Geometry: final body of the model. Coordinates: model frame, mm. Face numbers are marked on the shaded views. Give positions to 0.01 mm unless a question says otherwise; leave off trailing zeros. Write each loop counter-clockwise with the first axis right and the second up, starting at its lowest first coordinate (ties: lowest second). Pieces come first, ordered by that corner, then holes. Notation, with made-up numbers: (86, -13) - (132, -13) arc R28 ccw to (132, 17) - close; hole circle Ø2 at (4, 86.5). An arc over 180 degrees is marked (long way). Use CSV: the item, a comma, the result in double quotes. Start each with the question number.
(1) Section A-A on y = 0. Output: boundary loops of the cut face in (x, z), and give its area (3 significant figures).
(2) Section D-D on z = 87. Output: boundary loops of the cut face in (x, y).
(3) Section B-B on z = -21.5. Output: boundary loops of the cut face in (x, y).
(4) First-contact query: pin 1 Ø5 at (y, z) = (-79.5, -11.5) entering from -X; pin 2 Ø6 at (y, z) = (-25, 66.5) entering from +X; pin 3 Ø6 at (y, z) = (50, 42.5) entering from +X. Flat tips, straight axial feed; report the tip coordinate or a pass-through.
(5) Line query: probe 1 along Y at (x, z) = (0, -23); probe 2 along Y at (x, z) = (0, 63). Output: solid intervals per line, ascending. Write a range as [from, to].
(6) Draft query along Y for the marked faces 1, 2 and 3. Return one class per face: released by +Y, released by -Y, zero draft, split by the parting line, or undercut.
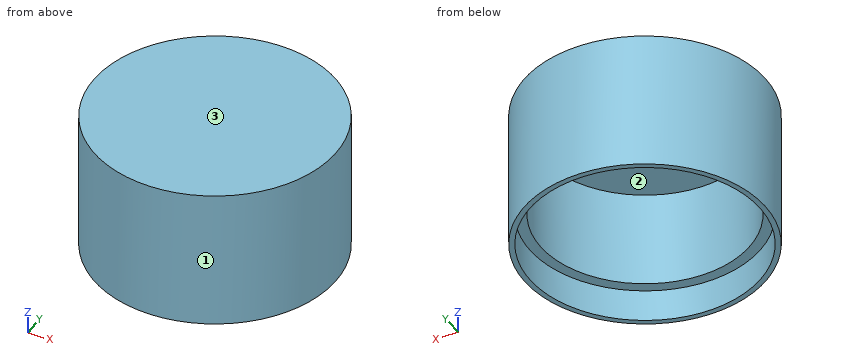
Autodesk Inventor part; units mm, degrees
ref_plane "YZ Plane" through (0, 0, 0) normal (1, 0, 0) x (0, 1, 0)
ref_plane "XZ Plane" through (0, 0, 0) normal (0, 1, 0) x (-1, 0, 0)
ref_plane "XY Plane" through (0, 0, 0) normal (0, 0, 1) x (1, 0, 0)
sketch "Sketch1" plane through (0, 0, 0) normal (1, 0, 0) x (0, 1, 0)
  line L0 (106.6, 0) -> (106.6, -254) construction
  line L1 (101.6, -254) -> (101.6, 0) construction
  line L2 (-106.6, 0) -> (106.6, 0) construction
  line L3 (107.1, 0) -> (107.1, -30)
  line L4 (107.1, -30) -> (112.1, -30)
  line L5 (112.1, -30) -> (112.1, 100)
  line L6 (112.1, 100) -> (0, 100)
  line L7 (107.1, 0) -> (97.1, 0)
  line L8 (97.1, 0) -> (97.1, 90)
  line L9 (97.1, 90) -> (0, 90)
  line L10 (0, 90) -> (0, 100)
  point P0 (0, 0)
  point P1 (0, 0)
  dimension "d2" = 5
  dimension "d4" = 0.5
  dimension "d5" = 30
  dimension "d6" = 100
  dimension "d8" = 10
  dimension "d9" = 10
revolve "Revolution1" add sketch "Sketch1" angle 360 about axis through (0, 0, 90) along (0, 0, 1)
properties part number "BackCapV1"
Check values:
1,outline,"(-112.1, -30) - (-107.1, -30) - (-107.1, 0) - (-97.1, 0) - (-97.1, 90) - (97.1, 90) - (97.1, 0) - (107.1, 0) - (107.1, -30) - (112.1, -30) - (112.1, 100) - (-112.1, 100) - close"
1,area,"5,240 mm²"
2,outline,"circle Ø224.2 at (0, 0); hole circle Ø194.2 at (0, 0)"
3,outline,"circle Ø224.2 at (0, 0); hole circle Ø214.2 at (0, 0)"
4,pin 1,"stops at x = -81.47"
4,pin 2,"stops at x = 109.92"
4,pin 3,"stops at x = 101.77"
5,probe 1,"y = [-112.1, -107.1], [107.1, 112.1]"
5,probe 2,"y = [-112.1, -97.1], [97.1, 112.1]"
6,face 1,"split by the parting line"
6,face 2,"undercut"
6,face 3,"zero draft"
